Read the model definition and answer for the solid it produces. Units are mm, in the model's axes. A direction names the side the tool comes from. Round coordinates to 2 decimals unless told otherwise and drop trailing zeros. Write each loop counter-clockwise with the first axis right and the second up, starting at its lowest first coordinate (ties: lowest second). Pieces come first, ordered by that corner, then holes. Notation, with made-up numbers: (-24.5, 67) -> (-20.5, 67) arc R16 ccw to (-20.5, 95) -> close; hole circle Ø10 at (-7, 84.5). An arc over 180 degrees is marked (long way). Return JSON: item names as keys, results as strings.
from build123d import *

# Parameters (mm, degrees)
CYLINDER004_R     = 7
CYLINDER004_DEPTH = 150
CYLINDER003_R     = 11
CYLINDER003_DEPTH = 31


with BuildPart() as axe:
    # Cylinder004 → Cylinder004 (new body)
    with BuildSketch(Plane.XY.offset(-50)):
        Circle(CYLINDER004_R)
    extrude(amount=CYLINDER004_DEPTH)


with BuildPart() as ball_slider:
    # Cylinder003 → Cylinder003 (new body)
    with BuildSketch(Plane.XY):
        Circle(CYLINDER003_R)
    extrude(amount=CYLINDER003_DEPTH)

    # Fusion003: union axe
    add(axe.part)


solid = ball_slider.part
Item 1: Section A-A (x = 0) is taken. Give the vertices of the cut face in (y, z).
Worked answers:
{"outline": "(-11, 0) -> (-7, 0) -> (-7, -50) -> (7, -50) -> (7, 0) -> (11, 0) -> (11, 31) -> (7, 31) -> (7, 100) -> (-7, 100) -> (-7, 31) -> (-11, 31) -> close"}
Item 2: Straight lines are drawn through the part: L1, parallel to Z at x = -8.5, y = -1; L2, parallel to Y at x = -0.5, z = 23.5; L3, parallel to Y at x = -0.25, z = 50.5. For each, find the intervals that lie inside material, in ascending order. Write a range as [from, to].
Worked answers:
{"L1": "z = [0, 31]", "L2": "y = [-10.99, 10.99]", "L3": "y = [-7, 7]"}
Item 3: Flat-ended cylindrical pins translate along their axes: pin 1 (12 mm diameter, centred on x = -6.5, z = 51, fed in from -Y); pin 2 (6 mm diameter, centred on x = 3.5, z = -23, fed in from +Y); pin 3 (4 mm diameter, centred on y = -2.5, z = 64, fed in from -X). Find the tip coordinate at first contact, or state that the pin passes through.
Worked answers:
{"pin 1": "stops at y = -6.98", "pin 2": "stops at y = 6.98", "pin 3": "stops at x = -6.98"}
Item 4: Section C-C (z = 8) is taken. Give the vertices of the cut face in (x, y).
Worked answers:
{"outline": "circle Ø22 at (0, 0)"}
Item 5: Section D-D (z = -20) is taken. Give the vertices of the cut face in (x, y).
Worked answers:
{"outline": "circle Ø14 at (0, 0)"}
Item 6: A tool of negligible diameter and unlimited length cuts with its end or side. For faces 1 (the flat face through (7.2, 0.2, 0)), 2 (the cylindrical face through (6.466, -2.681, 65.017)), 3 (the flat face through (0, 0, 100)), from which of +Z, -Z, +X, -X, +Y, -Y can it reach the whole face along a straight path? Write none if from no direction.
Worked answers:
{"face 1": "-Z", "face 2": "+Z", "face 3": "+Z, +X, -X, +Y, -Y"}
